from build123d import *

# Parameters (mm, degrees)
SKETCH1_R           = 3.7338
SKETCH1_R_2         = 2.6797
BOSS_EXTRUDE1_DEPTH = 1.1176
SHELL1_T            = -0.5715
BOSS_EXTRUDE2_DEPTH = 0.5588
SKETCH4_R           = 2.615046293
SKETCH4_R_2         = 2.107046293
BOSS_EXTRUDE3_DEPTH = 1.1176
BOSS_EXTRUDE4_DEPTH = 0.508


with BuildPart() as part:
    # Sketch1 → Boss-Extrude1 (new body)
    with BuildSketch(Plane(origin=(0, 0, 0), x_dir=(1, 0, 0), z_dir=(0, 1, 0))):
        with Locations(Location((0, 0, 0), (0, 0, 270))):
            Circle(SKETCH1_R)
        with Locations(Location((0, 0, 0), (0, 0, 270))):
            Circle(SKETCH1_R_2, mode=Mode.SUBTRACT)
    extrude(amount=-BOSS_EXTRUDE1_DEPTH)


with BuildPart() as body_2:
    # Sketch2 → Revolve1 (revolve)
    with BuildSketch(Plane.XY):
        with BuildLine():
            Line((0, -1.1176), (0, -20.9296))
            ThreePointArc((0, -20.9296), (-0.789505828, -20.640890822), (-1.206518449, -19.910977871))
            Line((-1.206518449, -19.910977871), (-2.770770199, -10.714786652))
            ThreePointArc((-2.770770199, -10.714786652), (-2.859495986, -10.068144543), (-2.906518408, -9.4171398))
            Line((-2.906518408, -9.4171398), (-3.2385, -1.1176))
            Line((-3.2385, -1.1176), (0, -1.1176))
        make_face()
    revolve(axis=Axis((0, -1.1176, 0), (0, -1, 0)))

    # Shell1
    shell1_openings = [body_2.faces().sort_by_distance(p)[0] for p in [
        (0, -1.1176, 0),
    ]]
    offset(amount=SHELL1_T, openings=shell1_openings, kind=Kind.INTERSECTION)


with BuildPart() as part_1:
    add(part.part)

    # Combine1: union body 2
    add(body_2.part)

    # Sketch3 → Boss-Extrude2 (add, symmetric)
    with BuildSketch(Plane.XY):
        with BuildLine():
            Line((3.7338, -1.1176), (4.365322861, -1.1176))
            Line((4.365322861, -1.1176), (5.180035681, -1.1176))
            ThreePointArc((5.180035681, -1.1176), (6.050241958, -0.247393722), (5.180035681, 0.622812555))
            Line((5.180035681, 0.622812555), (4.365322861, 0.622812555))
            Line((4.365322861, 0.622812555), (3.379294532, 0.622812555))
            Line((3.379294532, 0.622812555), (3.379294532, 0.112660745))
            Line((3.379294532, 0.112660745), (4.365322861, 0.112660745))
            Line((4.365322861, 0.112660745), (4.365322861, 0.36773665))
            Line((4.365322861, 0.36773665), (5.180035681, 0.36773665))
            ThreePointArc((5.180035681, 0.36773665), (5.795166053, -0.247393722), (5.180035681, -0.862524095))
            Line((5.180035681, -0.862524095), (4.365322861, -0.862524095))
            Line((4.365322861, -0.862524095), (4.365322861, -0.607448189))
            Line((4.365322861, -0.607448189), (3.379294532, -0.607448189))
            Line((3.379294532, -0.607448189), (3.379294532, -1.1176))
            Line((3.379294532, -1.1176), (3.7338, -1.1176))
        make_face()
    extrude(amount=BOSS_EXTRUDE2_DEPTH, both=True)



with BuildPart() as body_2_2:
    # Sketch4 → Boss-Extrude3 (new body)
    with BuildSketch(Plane.XZ.offset(-0.112660745)):
        with Locations(Location((0, 0, 0), (0, 0, 270))):
            Circle(SKETCH4_R)
        with Locations(Location((0, 0, 0), (0, 0, 270))):
            Circle(SKETCH4_R_2, mode=Mode.SUBTRACT)
    extrude(amount=BOSS_EXTRUDE3_DEPTH)


with BuildPart() as part_2:
    add(part_1.part)

    add(body_2_2.part)  # Boss-Extrude4 merges body 2 2
    # Sketch6 → Boss-Extrude4 (add)
    with BuildSketch(Plane.XZ.offset(-0.112660745)):
        with BuildLine():
            Line((-2.179935272, -3.062591525), (-4.50743423, -1.405890971))
            ThreePointArc((-4.50743423, -1.405890971), (-5.2324, 0), (-4.50743423, 1.405890971))
            Line((-4.50743423, 1.405890971), (-2.179935272, 3.062591525))
            ThreePointArc((-2.179935272, 3.062591525), (3.7592, 0), (-2.179935272, -3.062591525))
        make_face()
    extrude(amount=-BOSS_EXTRUDE4_DEPTH)


solid = part_2.part
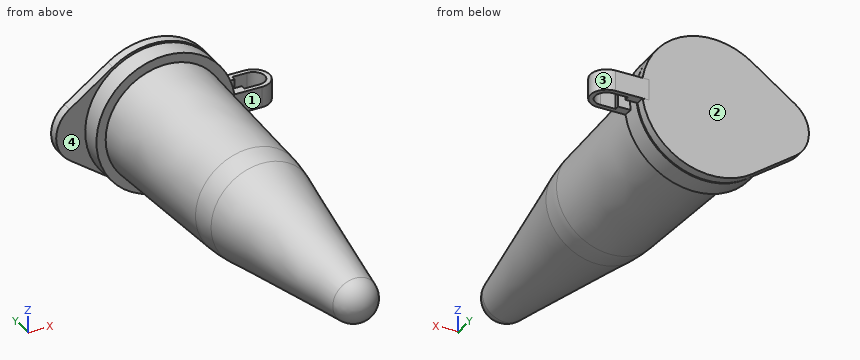
The model under review builds one solid part; all positions refer to its coordinate system, in mm. Face numbers are marked on the shaded views. Coordinates: 2 decimals unless noted, no trailing zeros. Order: outer loops, then holes, each group sorted by start corner. A loop starts at its lowest first (then second) coordinate and runs counter-clockwise, first axis right, second up. Notation, with made-up numbers: (-12.75, 7) -> (20.25, 7) arc R16 cw to (20.25, 21) -> close; hole circle Ø2 at (89.25, 52.25). An arc over 180 degrees is marked (long way). Answer in a Markdown table with one row per item.
(1) The part is to be moulded in two halves that separate along Y. For the marked faces 1, 2, 3 and 4, say which applies: +Y half, -Y half, draft (parallel to the pull), parting line (faces both ways), or undercut.
Answers:
| item | result |
|---|---|
| face 1 | -Y half |
| face 2 | +Y half |
| face 3 | parting line |
| face 4 | undercut |
(2) Consider section A-A (y = -2.25). Write out the cut boundary in (x, z).
Answers:
| item | result |
|---|---|
| outline | circle Ø6.39 at (0, 0); hole circle Ø5.24 at (0, 0) |
(3) Wall thickness on line 1 along X through (y, z) = (-9.25, -0.5); line 2 along X through (y, z) = (-6.5, 1); line 3 along Z through (x, y) = (-0.75, -13.5): over which ranges is each line inside the solid? List them lowest first.
Answers:
| item | result |
|---|---|
| line 1 | -2.87 to -2.29, 2.29 to 2.87 |
| line 2 | -2.85 to -2.24, 2.24 to 2.85 |
| line 3 | -2.17 to -1.54, 1.54 to 2.17 |
(4) Insertion check: pin 1 (4 mm diameter, centred on y = -15.5, z = 0.5, fed in from -X); pin 2 (4 mm diameter, centred on x = -2.5, z = -0.5, fed in from +Y); pin 3 (3.5 mm diameter, centred on x = -1.5, z = -2, fed in from -Y). Each pin has a flat end and moves straight along its axis. Give the tip position at first contact, or say it passes through.
Answers:
| item | result |
|---|---|
| pin 1 | x = -2.29 |
| pin 2 | y = 0.62 |
| pin 3 | y = -20.67 |
(5) Consider section B-B (y = -18). Write out the cut boundary in (x, z).
Answers:
| item | result |
|---|---|
| outline | circle Ø3.06 at (0, 0); hole circle Ø1.9 at (0, 0) |
